Job drawing, mm, ordinate dimensions from the low corner. One solid piece. Round coordinates to 2 decimals unless told otherwise and drop trailing zeros. Write each loop counter-clockwise with the first axis right and the second up, starting at its lowest first coordinate (ties: lowest second). Pieces come first, ordered by that corner, then holes.
1) Saw through at C-C (z = 0.45). Write the cut outline in (x, y).
2) Saw through at D-D (z = 3.15). Write the cut outline in (x, y), plus the area to 3 significant figures.
3) Wall check: probe 1 along Y at (x, z) = (4, 1.65); probe 2 along Y at (x, z) = (4, 1.1); probe 3 along X at (y, z) = (3, 1.9). Give the ranges that are in metal, low to high.
4) Pull direction X, two halves, no side cores. Call the marked faces 1, 2 and 3: +X half, -X half, draft (parallel to the pull), parting line (faces both ways), or undercut.
5) Flat gauge pins, fed straight in: pin 1 (2 mm diameter, centred on y = 6, z = 4.5, fed in from -X); pin 2 (1 mm diameter, centred on y = 4.5, z = 2.5, fed in from +X); pin 3 (2 mm diameter, centred on y = 6.5, z = 2, fed in from -X). Where does each tip first touch, or does it go through?
6) Saw through at A-A (y = 4). Write the cut outline in (x, z), plus the area to 3 significant figures.
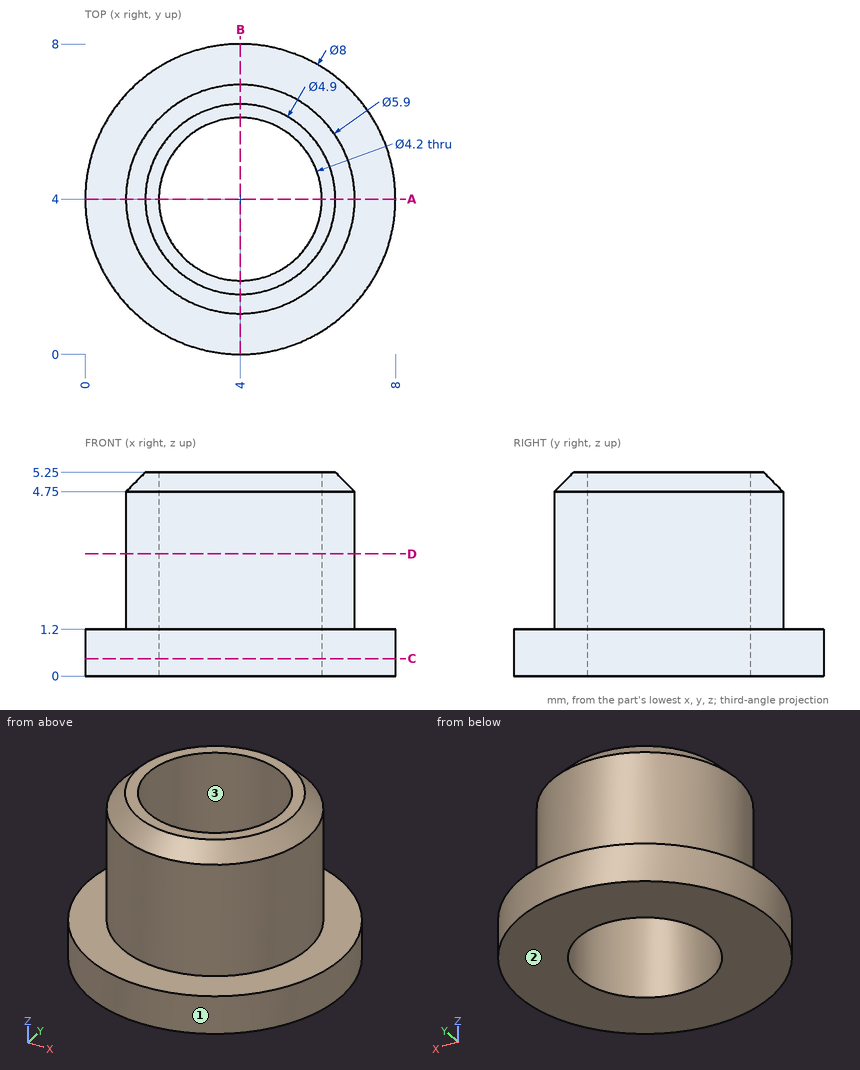
Evaluation:
1. outline: circle Ø8 at (4, 4); hole circle Ø4.2 at (4, 4)
2. outline: circle Ø5.9 at (4, 4); hole circle Ø4.2 at (4, 4)
2. area: 13.5 mm2
3. probe 1: y = 1.05 to 1.9, 6.1 to 6.95
3. probe 2: y = 0 to 1.9, 6.1 to 8
3. probe 3: x = 1.22 to 2.15, 5.85 to 6.78
4. face 1: parting line
4. face 2: draft
4. face 3: undercut
5. pin 1: stops at x = 1.22
5. pin 2: stops at x = 6.95
5. pin 3: stops at x = 0.48
6. outline: (0, 0) - (1.9, 0) - (1.9, 5.25) - (1.55, 5.25) - (1.05, 4.75) - (1.05, 1.2) - (0, 1.2) - close; (6.1, 0) - (8, 0) - (8, 1.2) - (6.95, 1.2) - (6.95, 4.75) - (6.45, 5.25) - (6.1, 5.25) - close
6. area: 11.2 mm2
